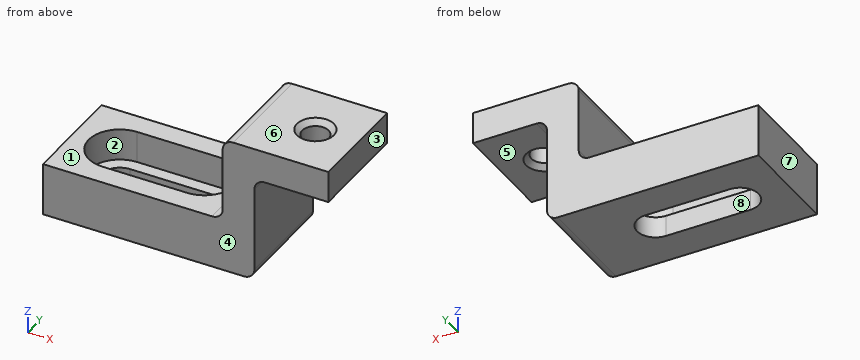
```python
from build123d import *

# Parameters (mm, degrees)
F0_W     = 17
F0_H     = 10
F1_DEPTH = 5
F2_DEPTH = 2
F3_W     = 10
F3_H     = 10
F4_DEPTH = 3
F5_W     = 10
F5_H     = 10
F5_R     = 1.25
F6_DEPTH = 3
F7_R     = 1
F8_SIZE  = 0.5


with BuildPart() as f1:
    # F0 (on Top) → F1 (new body)
    with BuildSketch(Plane.XY):
        Rectangle(F0_W, F0_H)
        with BuildLine():
            ThreePointArc((-4, -2.95), (-6.95, 0), (-4, 2.95))
            Line((-4, 2.95), (4, 2.95))
            ThreePointArc((4, 2.95), (6.0859650045, 2.0859650045), (6.95, 0))
            ThreePointArc((6.95, 0), (6.0859650045, -2.0859650045), (4, -2.95))
            Line((4, -2.95), (-4, -2.95))
        make_face(mode=Mode.SUBTRACT)
    extrude(amount=F1_DEPTH)

    # F0 (on Top) → F2 (join)
    with BuildSketch(Plane.XY):
        with BuildLine():
            ThreePointArc((-4, -1.75), (-5.75, 0), (-4, 1.75))
            Line((-4, 1.75), (-4, 2.95))
            ThreePointArc((-4, 2.95), (-6.95, 0), (-4, -2.95))
            Line((-4, -2.95), (-4, -1.75))
        make_face()
        with BuildLine():
            Line((-4, 2.95), (-4, 1.75))
            Line((-4, 1.75), (-1.6251315826, 1.75))
            ThreePointArc((-1.6251315826, 1.75), (-2.6695865304, 2.6329641091), (-4, 2.95))
        make_face()
        with BuildLine():
            ThreePointArc((-4, 2.95), (-2.6695865304, 2.6329641091), (-1.6251315826, 1.75))
            Line((-1.6251315826, 1.75), (1.6251315826, 1.75))
            ThreePointArc((1.6251315826, 1.75), (2.6695865304, 2.6329641091), (4, 2.95))
            Line((4, 2.95), (-4, 2.95))
        make_face()
        with BuildLine():
            ThreePointArc((4, 2.95), (2.6695865304, 2.6329641091), (1.6251315826, 1.75))
            Line((1.6251315826, 1.75), (4, 1.75))
            Line((4, 1.75), (4, 2.95))
        make_face()
        with BuildLine():
            ThreePointArc((6.95, 0), (6.0859650045, 2.0859650045), (4, 2.95))
            Line((4, 2.95), (4, 1.75))
            ThreePointArc((4, 1.75), (5.2374368671, 1.2374368671), (5.75, 0))
            ThreePointArc((5.75, 0), (5.2374368671, -1.2374368671), (4, -1.75))
            Line((4, -1.75), (4, -2.95))
            ThreePointArc((4, -2.95), (6.0859650045, -2.0859650045), (6.95, 0))
        make_face()
        with BuildLine():
            Line((4, -1.75), (1.6251315826, -1.75))
            ThreePointArc((1.6251315826, -1.75), (2.6695865304, -2.6329641091), (4, -2.95))
            Line((4, -2.95), (4, -1.75))
        make_face()
        with BuildLine():
            Line((1.6251315826, -1.75), (-1.6251315826, -1.75))
            ThreePointArc((-1.6251315826, -1.75), (-2.6695865304, -2.6329641091), (-4, -2.95))
            Line((-4, -2.95), (4, -2.95))
            ThreePointArc((4, -2.95), (2.6695865304, -2.6329641091), (1.6251315826, -1.75))
        make_face()
        with BuildLine():
            Line((-1.6251315826, -1.75), (-4, -1.75))
            Line((-4, -1.75), (-4, -2.95))
            ThreePointArc((-4, -2.95), (-2.6695865304, -2.6329641091), (-1.6251315826, -1.75))
        make_face()
    extrude(amount=F2_DEPTH)

    # F3 (on face) → F4 (join)
    with BuildSketch(Plane.YZ.offset(8.5)):
        with Locations((0, 5)):
            Rectangle(F3_W, F3_H)
    extrude(amount=F4_DEPTH)

    # F5 (on face) → F6 (join)
    with BuildSketch(Plane.XY.offset(10)):
        with Locations((13.5, 0)):
            Rectangle(F5_W, F5_H)
        with Locations((14.5, 0)):
            Circle(F5_R, mode=Mode.SUBTRACT)
    extrude(amount=F6_DEPTH)

    # F7
    f7_edges = [f1.edges().sort_by_distance(p)[0] for p in [
        (8.5, 0, 13),
        (11.5, 0, 10),
        (11.5, 0, 0),
        (8.5, 0, 5),
    ]]
    fillet(f7_edges, radius=F7_R)

    # F8
    f8_edges = [f1.edges().sort_by_distance(p)[0] for p in [
        (15.75, 0, 11.5),
        (13.25, 0, 10),
        (13.25, 0, 13),
    ]]
    chamfer(f8_edges, length=F8_SIZE)


solid = f1.part
```
Source: CAD feature listing. Evaluate the final solid. Frame: model axes, mm. Face numbers are marked on the shaded views. A direction names the side the tool comes from. Coordinates: 2 decimals unless noted, no trailing zeros. Loops run counter-clockwise (first coordinate to the right, second up) from the corner with the lowest first, then second, coordinate; pieces in that order, holes last. Notation, with made-up numbers: M 54.25,73 L 69.25,73 A18 cw 69.25,93 Z; hole C -0.5,-26 d10. An arc over 180 degrees is marked long. Put each result on its own line as item: value. Start each with the question number.
1) Ray query, L1, parallel to Y at x = 14.5, z = 11.05; L2, parallel to Y at x = -4, z = 3; L3, parallel to Z at x = -1.5, y = 2.5. Return the intervals inside material, ascending. Write a range as from..to.
2) Cut plane C-C on y = 4. Return the cut outline in (x, z).
3) Reachability of the marked faces 1, 2, 3, 4 and 5 from +Z, -Z, +X, -X, +Y, -Y: full face, straight path, thin tool, end or side. Return the list, or none.
4) Cut plane B-B on z = 4.5. Return the cut outline in (x, y), then the cut area to 3 significant figures.
5) Contact query for flat-ended pins moving along their axis: pin 1 Ø4 at (y, z) = (0, 3.5) entering from +X; pin 2 Ø1.5 at (x, y) = (-4, 4) entering from +Z; pin 3 Ø3 at (x, y) = (1.5, 0) entering from +Z; pin 4 Ø3 at (x, y) = (14.5, -2.5) entering from -Z. Output: stop coordinate, or through.
6) Pull-direction query (X, two-part tool) for the marked faces 6, 7 and 8; classes: pulls with the +X half, pulls with the -X half, needs draft (parallel to the pull), parting line crosses it, or undercut.
7) Cut plane D-D on x = 14.5. Return the cut outline in (y, z), then the cut area to 3 significant figures.
8) Cut plane A-A on x = 2.75. Return the cut outline in (y, z).
The answers:
1. L1: y = -5..-1.25, 1.25..5
1. L2: y = -5..-2.95, 2.95..5
1. L3: z = 0..2
2. outline: M -8.5,0 L 10.5,0 A1 ccw 11.5,1 L 11.5,9 A1 cw 12.5,10 L 18.5,10 L 18.5,13 L 9.5,13 A1 ccw 8.5,12 L 8.5,6 A1 cw 7.5,5 L -8.5,5 Z
3. face 1: +Z, -X, +Y, -Y
3. face 2: +Z
3. face 3: +Z, -Z, +X, +Y, -Y
3. face 4: +Z, -Z, +X, -X, -Y
3. face 5: -Z, +X, +Y, -Y
4. outline: M -8.5,-5 L 11.5,-5 L 11.5,5 L -8.5,5 Z; hole M -4,-2.95 L 4,-2.95 A2.95 ccw 4,2.95 L -4,2.95 A2.95 ccw Z
4. area: 125 mm²
5. pin 1: stops at x = 11.5
5. pin 2: stops at z = 5
5. pin 3: passes through
5. pin 4: stops at z = 10
6. face 6: needs draft
6. face 7: pulls with the -X half
6. face 8: undercut
7. outline: M -5,10 L -1.75,10 L -1.25,10.5 L -1.25,12.5 L -1.75,13 L -5,13 Z; M 1.25,10.5 L 1.75,10 L 5,10 L 5,13 L 1.75,13 L 1.25,12.5 Z
7. area: 22.0 mm²
8. outline: M -5,0 L -1.75,0 L -1.75,2 L -2.95,2 L -2.95,5 L -5,5 Z; M 1.75,0 L 5,0 L 5,5 L 2.95,5 L 2.95,2 L 1.75,2 Z
